Read the model definition and answer for the solid it produces. Units are mm, in the model's axes. A direction names the side the tool comes from. Give positions to 0.01 mm unless a question says otherwise; leave off trailing zeros. Order: outer loops, then holes, each group sorted by start corner. A loop starts at its lowest first (then second) coordinate and runs counter-clockwise, first axis right, second up. Notation, with made-up numbers: (-5, -28) - (39, -28) arc R28 ccw to (39, 0) - close; hole circle Ø10 at (72, 57). An arc over 180 degrees is marked (long way). Write item = value, one per line.
```python
from build123d import *

# Parameters (mm, degrees)
BOSS_EXTRUDE1_DEPTH = 30
SKETCH2_R           = 11
BOSS_EXTRUDE2_DEPTH = 45
SKETCH3_R           = 7.5
CUT_EXTRUDE1_DEPTH  = 5
CUT_EXTRUDE2_START  = -5
SKETCH4_R           = 7.5
CUT_EXTRUDE2_DEPTH  = 5


with BuildPart() as part:
    # Sketch1 → Boss-Extrude1 (new body)
    with BuildSketch(Plane.XY):
        Polygon((164.243144092, -242.240505044), (107.282313119, -242.240505044), (107.282313119, -269.240505044), (245.890540796, -269.240505044), (245.890540796, -27.289352142), (247.838560611, -26.297684258), (247.838560611, -18.825937148), (245.890540796, -17.450821047), (245.890540796, -13.240505044), (236.499007707, -13.240505044), (226.537313119, -0.206413948), (226.537313119, -32.526046634), (235.73808569, -27.842259234), (235.73808569, -242.240505044), (222.507031976, -242.240505044), (212.571392529, -255.240505044), (174.178783539, -255.240505044), align=None)
        Polygon((107.282313119, -242.240505044), (50.321482145, -242.240505044), (40.385842698, -255.240505044), (1.993233708, -255.240505044), (-7.942405739, -242.240505044), (-21.173459453, -242.240505044), (-21.173459453, -27.842259234), (-11.972686881, -32.526046634), (-11.972686881, -0.206413948), (-21.93438147, -13.240505044), (-31.325914559, -13.240505044), (-31.325914559, -17.450821047), (-33.273934374, -18.825937148), (-33.273934374, -26.297684258), (-31.325914559, -27.289352142), (-31.325914559, -269.240505044), (107.282313119, -269.240505044), align=None)
    extrude(amount=BOSS_EXTRUDE1_DEPTH)

    # Sketch2 → Boss-Extrude2 (add)
    with BuildSketch(Plane.XZ.offset(269.240505044)):
        with Locations(Location((107.282313119, 15, 0), (0, 0, 90))):
            Circle(SKETCH2_R)
    extrude(amount=BOSS_EXTRUDE2_DEPTH)

    # Sketch3 → Cut-Extrude1 (cut)
    with BuildSketch(Plane(origin=(-11.972686881, 0, 0), x_dir=(0, 0, -1), z_dir=(1, 0, 0))):
        with Locations((-15, -16.366230291)):
            Circle(SKETCH3_R)
    extrude(amount=-CUT_EXTRUDE1_DEPTH, mode=Mode.SUBTRACT)

    # Sketch4 → Cut-Extrude2 (cut)
    with BuildSketch(Plane.ZY.offset(-226.537313119).offset(CUT_EXTRUDE2_START)):
        with Locations(Location((15, -16.366230291, 0), (0, 0, 180))):
            Circle(SKETCH4_R)
    extrude(amount=CUT_EXTRUDE2_DEPTH, mode=Mode.SUBTRACT)


solid = part.part
```
1. Flat-ended cylindrical pins translate along their axes: pin 1 (12 mm diameter, centred on y = -16.37, z = 15, fed in from +X); pin 2 (9 mm diameter, centred on y = -155, z = 19, fed in from +X); pin 3 (6.5 mm diameter, centred on x = 227.5, z = 13.5, fed in from +Y); pin 4 (1.5 mm diameter, centred on y = -281.5, z = 9.5, fed in from +X). Find the tip coordinate at first contact, or state that the pin passes through.
Recorded:
pin_1 = 247.84
pin_2 = 245.89
pin_3 = -0.21
pin_4 = 117.2
2. For faces 4 (the face through (245.891, -150, 15)), 5 (the face through (-11.973, -20, 8)), 6 (the face through (231.537, -16, 15)), determine the directions among +Z, -Z, +X, -X, +Y, -Y from which every point of the face is accessible in a straight line to the end or side of a thin tool.
Recorded:
face_4 = +Z, -Z, +X, -Y
face_5 = +Z, -Z, +Y
face_6 = none
3. Determine the mould class of faces 1 (the face through (231.07, -30.22, 14.79)), 2 (the face through (-31.326, -147, 15)), 3 (the face through (217.61, -248.65, 14.79)) for opening direction Y: +Y half, -Y half, draft (parallel to the pull), parting line (faces both ways), or undercut.
Recorded:
face_1 = undercut
face_2 = draft
face_3 = +Y half
4. Straight lines are drawn through the part: L1, parallel to X at y = -19.5, z = 24; L2, parallel to X at y = -86.5, z = 12.5; L3, parallel to Y at x = -14.5, z = 15. For each, find the intervals that lie inside material, in ascending order. Write a range as [from, to].
Recorded:
L1 = [-33.27, -11.97], [226.54, 247.84]
L2 = [-31.33, -21.17], [235.74, 245.89]
L3 = [-269.24, -242.24], [-31.24, -23.87], [-8.87, -3.51]
5. Section B-B (x = 15.5) is taken. Determine the outline of the cut face in (y, z).
Recorded:
outline = (-269.24, 0) - (-255.24, 0) - (-255.24, 30) - (-269.24, 30) - close
6. Section A-A (y = -111.5) is taken. Determine the outline of the cut face in (x, z).
Recorded:
outline = (-31.33, 0) - (-21.17, 0) - (-21.17, 30) - (-31.33, 30) - close; (235.74, 0) - (245.89, 0) - (245.89, 30) - (235.74, 30) - close
7. Section C-C (x = 76.5) is taken. Determine the outline of the cut face in (y, z), and give its area (3 significant figures).
Recorded:
outline = (-269.24, 0) - (-242.24, 0) - (-242.24, 30) - (-269.24, 30) - close
area = 810 mm^2
